Study the drawing (mm; zero at the part's minimum x, y, z) and answer. Round coordinates to 2 decimals unless told otherwise and drop trailing zeros. Loops run counter-clockwise (first coordinate to the right, second up) from the corner with the lowest first, then second, coordinate; pieces in that order, holes last. Notation, with made-up numbers: (-3.75, 52) -> (31.25, 52) arc R23 cw to (31.25, 89) -> close; hole circle Ø4 at (14, -18). An arc over 180 degrees is marked (long way). Write each question's results on one line, items separated by ' | '. Start each with the question number.
(1) The part is cut by section B-B (y = 35). Determine the outline of the cut face in (x, z), plus the area to 3 significant figures.
(2) The part is cut by section A-A (x = 86.5). Determine the outline of the cut face in (y, z).
(3) The part is cut by section C-C (z = 1.4). Count the separate pieces of the cut face and the enclosed holes in it, plus the area to 3 significant figures.
(4) A flat-ended cylindrical pin translates along its axis: pin 1 (0.9 mm diameter, centred on x = 68, z = 2, fed in from -Y). Find the tip coordinate at first contact, or state that the pin passes through.
(5) Straight lines are drawn through the part: probe 1 along Y at (x, z) = (42.5, 0.55); probe 2 along Y at (x, z) = (74.5, 0.2); probe 3 along X at (y, z) = (15, 0.65). For each, find the intervals that lie inside material, in ascending order.
(6) The part is cut by section D-D (y = 25). Determine the outline of the cut face in (x, z).
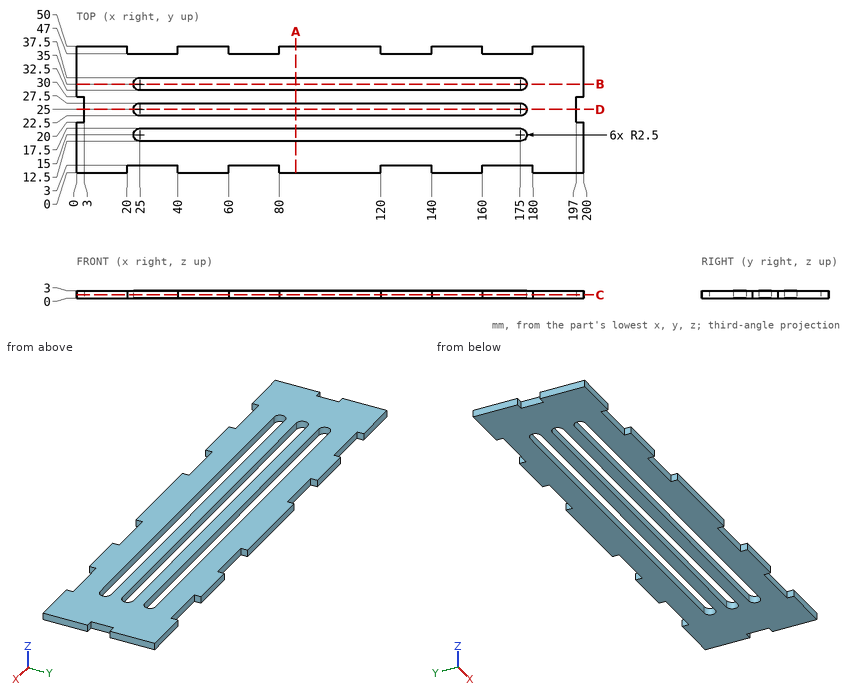
Checked values:
1) outline: (0, 0) -> (22.5, 0) -> (22.5, 3) -> (0, 3) -> close; (177.5, 0) -> (200, 0) -> (200, 3) -> (177.5, 3) -> close | area: 135 mm2
2) outline: (0, 0) -> (12.5, 0) -> (12.5, 3) -> (0, 3) -> close; (17.5, 0) -> (22.5, 0) -> (22.5, 3) -> (17.5, 3) -> close; (27.5, 0) -> (32.5, 0) -> (32.5, 3) -> (27.5, 3) -> close; (37.5, 0) -> (50, 0) -> (50, 3) -> (37.5, 3) -> close
3) separate pieces: 1 | enclosed holes: 3 | area: 7,150 mm2
4) pin 1: stops at y = 3
5) probe 1: y = 0 to 12.5, 17.5 to 22.5, 27.5 to 32.5, 37.5 to 50 | probe 2: y = 3 to 12.5, 17.5 to 22.5, 27.5 to 32.5, 37.5 to 47 | probe 3: x = 0 to 22.5, 177.5 to 200
6) outline: (3, 0) -> (22.5, 0) -> (22.5, 3) -> (3, 3) -> close; (177.5, 0) -> (197, 0) -> (197, 3) -> (177.5, 3) -> close
